Read the model definition and answer for the solid it produces. Units are mm, in the model's axes. A direction names the side the tool comes from. Coordinates: 2 decimals unless noted, no trailing zeros. Write each loop counter-clockwise with the first axis right and the second up, starting at its lowest first coordinate (ties: lowest second). Pieces come first, ordered by that corner, then holes. Notation, with made-up numbers: (43.25, 72) -> (69.25, 72) arc R18 cw to (69.25, 80) -> close; hole circle Ø5 at (28, 16). An arc over 180 degrees is marked (long way). One line per item, written item: value. Start each with the question number.
1. Find section C-C, the plane z = -124. Write down the section's boundary in (x, y), and give its area (3 significant figures).
2. Find section B-B, the plane x = 14.25. State how many separate pieces and enclosed holes the cut face has, and give its area (3 significant figures).
3. For faces 5 (the flat face through (13, -107.019, 3)), 6 (the flat face through (13, -146, -114.3)), 7 (the flat face through (13, -143, -222.25)), 8 (the flat face through (13, -83, -8.4)), determine the directions among +Z, -Z, +X, -X, +Y, -Y from which every point of the face is accessible in a straight line to the end or side of a thin tool.
4. Given P1, Ø3, axis at x = 11.5, y = -146.5, coming from the +Z side; P2, Ø1.9, axis at x = 13.5, y = -146.5, coming from the -Z side; P3, Ø1.9, axis at x = 13.5, y = -84, coming from the +Z side, each flat-ended and moving along its own axis, determine where each tip first touches the part or whether it passes through.
5. For a pull along Z with two mould halves and no side action, classify faces 1 (the flat face through (13, -143.002, -94)), 2 (the flat face through (13, -98, 6.35)), 3 (the flat face through (13, -149.352, -189)), 4 (the flat face through (13, -146, -155.575)) as pulls with the +Z half, pulls with the -Z half, needs draft (parallel to the pull), parting line crosses it, or undercut.
6. Consider line 1 along Z through (x, y) = (13.75, -80); line 2 along Y through (x, z) = (11.75, -173); line 3 along Y through (x, z) = (15, -40.5). Determine where each line is inside the solid, lowest interval first.
7. Find section A-A, the plane z = -25.4. Write down the section's boundary in (x, y).
```python
from build123d import *

# Parameters (mm, degrees)
SKETCH1_W               = 44.958
SKETCH1_H               = 304.8
BOSS_EXTRUDE1_DEPTH     = 6.35
SKETCH2_W               = 6.35
SKETCH2_H               = 101.6
BOSS_EXTRUDE2_DEPTH     = 6.35
SKETCH3_W               = 222.25
SKETCH3_H               = 6.35
BOSS_EXTRUDE3_DEPTH     = 38.608
SKETCH8_W               = 6.35
SKETCH8_H               = 213.451350416
CUT_EXTRUDE4_DEPTH      = 1
CUT_EXTRUDE4_DEPTH_BACK = 235.95
SKETCH6_W               = 6.35
SKETCH6_H               = 12.7
CUT_EXTRUDE5_DEPTH      = 6.35
SKETCH4_3_W             = 6.35
SKETCH4_3_H             = 14.2875
SKETCH4_3_H_2           = 6.35
CUT_EXTRUDE6_DEPTH      = 6.35


with BuildPart() as part:
    # Sketch1 → Boss-Extrude1 (new body)
    with BuildSketch(Plane.XY):
        with Locations((-6.477, 3.048)):
            Rectangle(SKETCH1_W, SKETCH1_H)
        with BuildLine():
            Line((-3.302, 133.858), (-3.302, -143.002))
            Line((-3.302, -143.002), (3.302, -143.002))
            Line((3.302, -143.002), (3.302, 143.002))
            Line((3.302, 143.002), (-16.256, 143.002))
            Line((-16.256, 143.002), (-16.256, 136.398))
            Line((-16.256, 136.398), (-5.842, 136.398))
            ThreePointArc((-5.842, 136.398), (-4.045948776, 135.654051224), (-3.302, 133.858))
        make_face(mode=Mode.SUBTRACT)
    extrude(amount=BOSS_EXTRUDE1_DEPTH)

    # Sketch2 → Boss-Extrude2 (add)
    with BuildSketch(Plane(origin=(16.002, 0, 0), x_dir=(0, 0, -1), z_dir=(1, 0, 0))):
        Polygon((222.25, -60.452), (222.25, -47.752), (0, -47.752), (0, -149.352), (222.25, -149.352), (222.25, -136.652), (228.6, -136.652), (228.6, -119.718666667), (222.25, -119.718666667), (222.25, -107.018666667), (228.6, -107.018666667), (228.6, -90.085333333), (222.25, -90.085333333), (222.25, -77.385333333), (228.6, -77.385333333), (228.6, -60.452), align=None)
        with BuildLine():
            ThreePointArc((11.4, -116.592), (9.9, -118.092), (8.4, -116.592))
            Line((8.4, -116.592), (8.4, -111.512))
            ThreePointArc((8.4, -111.512), (9.9, -110.012), (11.4, -111.512))
            Line((11.4, -111.512), (11.4, -116.592))
        make_face(mode=Mode.SUBTRACT)
        with BuildLine():
            Line((42.4, -111.512), (42.4, -116.592))
            ThreePointArc((42.4, -116.592), (40.9, -118.092), (39.4, -116.592))
            Line((39.4, -116.592), (39.4, -111.512))
            ThreePointArc((39.4, -111.512), (40.9, -110.012), (42.4, -111.512))
        make_face(mode=Mode.SUBTRACT)
        with BuildLine():
            ThreePointArc((36.4, -101.092), (25.4, -112.092), (14.4, -101.092))
            Line((14.4, -101.092), (14.4, -96.012))
            ThreePointArc((14.4, -96.012), (25.4, -85.012), (36.4, -96.012))
            Line((36.4, -96.012), (36.4, -101.092))
        make_face(mode=Mode.SUBTRACT)
        with BuildLine():
            ThreePointArc((11.4, -85.592), (9.9, -87.092), (8.4, -85.592))
            Line((8.4, -85.592), (8.4, -80.512))
            ThreePointArc((8.4, -80.512), (9.9, -79.012), (11.4, -80.512))
            Line((11.4, -80.512), (11.4, -85.592))
        make_face(mode=Mode.SUBTRACT)
        with BuildLine():
            ThreePointArc((42.4, -85.592), (40.9, -87.092), (39.4, -85.592))
            Line((39.4, -85.592), (39.4, -80.512))
            ThreePointArc((39.4, -80.512), (40.9, -79.012), (42.4, -80.512))
            Line((42.4, -80.512), (42.4, -85.592))
        make_face(mode=Mode.SUBTRACT)
        with Locations((-3.175, -98.552)):
            Rectangle(SKETCH2_W, SKETCH2_H)
    extrude(amount=-BOSS_EXTRUDE2_DEPTH)

    # Sketch3 → Boss-Extrude3 (add)
    with BuildSketch(Plane.ZY.offset(-9.652)):
        with Locations((-111.125, -146.177)):
            Rectangle(SKETCH3_W, SKETCH3_H)
    extrude(amount=BOSS_EXTRUDE3_DEPTH)

    # Sketch8 → Cut-Extrude4 (cut, two sides)
    with BuildSketch(Plane.XY.offset(6.35)) as cut_extrude4_sk:
        Polygon((-28.956, -149.352), (9.652, -149.352), (9.652, -47.752), (9.652, 155.448), (-28.956, 155.448), align=None)
        with BuildLine():
            Line((-16.256, 136.398), (-16.256, 143.002))
            Line((-16.256, 143.002), (3.302, 143.002))
            Line((3.302, 143.002), (3.302, -143.002))
            Line((3.302, -143.002), (-3.302, -143.002))
            Line((-3.302, -143.002), (-3.302, 133.858))
            ThreePointArc((-3.302, 133.858), (-4.045948776, 135.654051224), (-5.842, 136.398))
            Line((-5.842, 136.398), (-16.256, 136.398))
        make_face(mode=Mode.SUBTRACT)
        Polygon((-54.223542679, -149.352), (-28.956, -149.352), (-28.956, 155.448), (9.652, 155.448), (9.652, 165.699350416), (-54.223542679, 165.699350416), align=None)
        with Locations((12.827, 58.973675208)):
            Rectangle(SKETCH8_W, SKETCH8_H)
    extrude(amount=CUT_EXTRUDE4_DEPTH, mode=Mode.SUBTRACT)
    extrude(cut_extrude4_sk.sketch, amount=-CUT_EXTRUDE4_DEPTH_BACK, mode=Mode.SUBTRACT)

    # Sketch6 → Cut-Extrude5 (cut)
    with BuildSketch(Plane.XY.offset(6.35)):
        with Locations((12.827, -54.102)):
            Rectangle(SKETCH6_W, SKETCH6_H)
        with Locations((12.827, -83.735333333)):
            Rectangle(SKETCH6_W, SKETCH6_H)
        with Locations((12.827, -113.368666667)):
            Rectangle(SKETCH6_W, SKETCH6_H)
        with Locations((12.827, -143.002)):
            Rectangle(SKETCH6_W, SKETCH6_H)
    extrude(amount=-CUT_EXTRUDE5_DEPTH, mode=Mode.SUBTRACT)

    # Sketch4<3> → Cut-Extrude6 (cut)
    with BuildSketch(Plane.XZ.offset(149.352)):
        with Locations((12.827, -13.49375)):
            Rectangle(SKETCH4_3_W, SKETCH4_3_H)
        with Locations((12.827, -40.48125)):
            Rectangle(SKETCH4_3_W, SKETCH4_3_H)
        with Locations((12.827, -67.46875)):
            Rectangle(SKETCH4_3_W, SKETCH4_3_H)
        with Locations((12.827, -94.45625)):
            Rectangle(SKETCH4_3_W, SKETCH4_3_H)
        with Locations((12.827, -121.44375)):
            Rectangle(SKETCH4_3_W, SKETCH4_3_H)
        with Locations((12.827, -148.43125)):
            Rectangle(SKETCH4_3_W, SKETCH4_3_H)
        with Locations((12.827, -175.41875)):
            Rectangle(SKETCH4_3_W, SKETCH4_3_H)
        with Locations((12.827, -202.40625)):
            Rectangle(SKETCH4_3_W, SKETCH4_3_H)
        with Locations((12.827, -3.175)):
            Rectangle(SKETCH4_3_W, SKETCH4_3_H_2)
        with Locations((12.827, 3.175)):
            Rectangle(SKETCH4_3_W, SKETCH4_3_H_2)
    extrude(amount=-CUT_EXTRUDE6_DEPTH, mode=Mode.SUBTRACT)


solid = part.part
```
Answer block:
1. outline: (9.65, -143) -> (16, -143) -> (16, -47.75) -> (9.65, -47.75) -> close
1. area: 605 mm2
2. separate pieces: 1
2. enclosed holes: 5
2. area: 21,900 mm2
3. face 5: +Z, +X, -X
3. face 6: +X, -X, -Y
3. face 7: -Z, +X, -X, -Y
3. face 8: +X, -X
4. P1: stops at z = -20.64
4. P2: stops at z = -222.25
4. P3: stops at z = 0
5. face 1: undercut
5. face 2: pulls with the +Z half
5. face 3: needs draft
5. face 4: undercut
6. line 1: z = -222.25 to -42.31, -39.49 to -11.31, -8.49 to 0
6. line 2: y = -143 to -47.75
6. line 3: y = -143 to -118.04, -110.07 to -87.04, -79.07 to -47.75
7. outline: (9.65, -149.35) -> (16, -149.35) -> (16, -112.09) -> (9.65, -112.09) -> close; (9.65, -85.01) -> (16, -85.01) -> (16, -47.75) -> (9.65, -47.75) -> close
